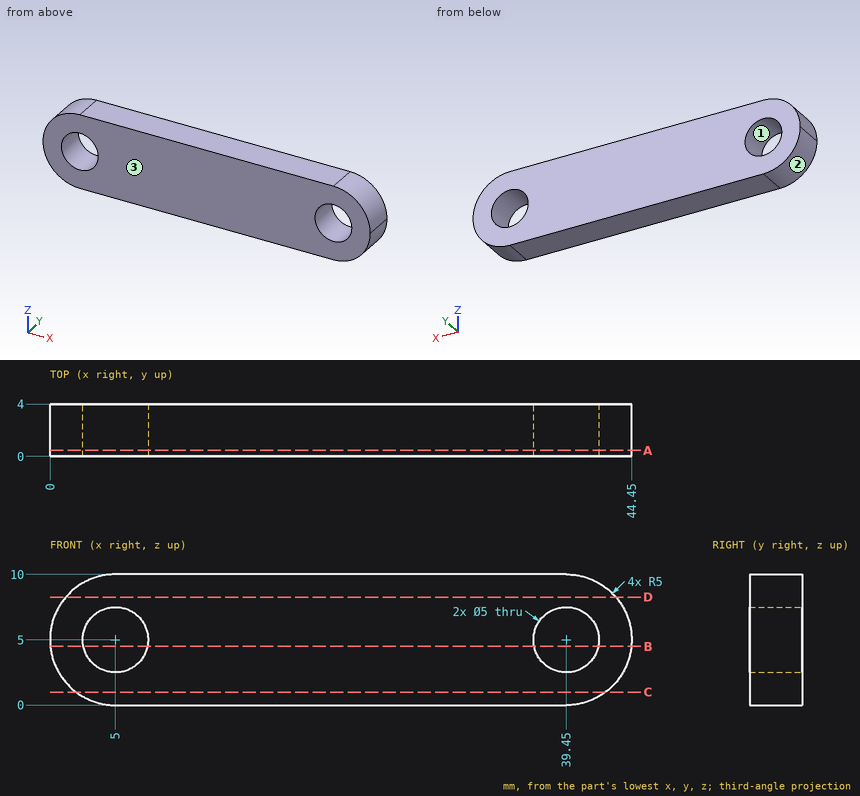
Can you work these out from the drawing? Everything is in mm from the part's minimum corner. Coordinates: 2 decimals unless noted, no trailing zeros. Loops run counter-clockwise (first coordinate to the right, second up) from the corner with the lowest first, then second, coordinate; pieces in that order, holes last.
1. Imagine slicing it at D-D, the plane z = 8.25. Please give me the cut outline in (x, y).
2. For P1, Ø1, axis at y = 2, z = 2, coming from the -X side; P2, Ø1.5, axis at y = 2.5, z = 2.5, coming from the +X side, each with a flat end and sliding along its axis, tell me the tip position at first contact or that it passes through.
3. Imagine slicing it at B-B, the plane z = 4.5. Please give me the cut outline in (x, y) (1 decimal).
4. If we mould it in two halves opening along X, with no side actions, what happens to the marked faces 1, 2 and 3? For each: pulls with the +X half, pulls with the -X half, needs draft (parallel to the pull), parting line crosses it, or undercut.
5. Imagine slicing it at A-A, the plane y = 0.45. Count the separate pieces of the cut face and the enclosed holes in it, and give its area (3 significant figures).
6. I need wall thicknesses on L1, parallel to X at y = 2.5, z = 5; L2, parallel to Z at x = 39.45, y = 1.1; L3, parallel to X at y = 3.25, z = 6.5. Which ranges of each line are inside material? Lowest first, please.
7. Imagine slicing it at C-C, the plane z = 1. Please give me the cut outline in (x, y).
Taken from the geometry:
1. outline: (1.2, 0) - (43.25, 0) - (43.25, 4) - (1.2, 4) - close
2. P1: stops at x = 0.67
2. P2: stops at x = 44.13
3. outline: (0, 0) - (2.6, 0) - (2.6, 4) - (0, 4) - close; (7.4, 0) - (37, 0) - (37, 4) - (7.4, 4) - close; (41.9, 0) - (44.4, 0) - (44.4, 4) - (41.9, 4) - close
4. face 1: undercut
4. face 2: pulls with the -X half
4. face 3: needs draft
5. separate pieces: 1
5. enclosed holes: 2
5. area: 384 mm2
6. L1: x = 0 to 2.5, 7.5 to 36.95, 41.95 to 44.45
6. L2: z = 0 to 2.5, 7.5 to 10
6. L3: x = 0.23 to 3, 7 to 37.45, 41.45 to 44.22
7. outline: (2, 0) - (42.45, 0) - (42.45, 4) - (2, 4) - close
